Work out the finished part from the listing and answer in its coordinate system (mm). Coordinates: 2 decimals unless noted, no trailing zeros. Order: outer loops, then holes, each group sorted by start corner. A loop starts at its lowest first (then second) coordinate and runs counter-clockwise, first axis right, second up.
1. Flat-ended cylindrical pins translate along their axes: pin 1 Ø0.6 at (x, y) = (-1, -14) entering from -Z; pin 2 Ø1 at (x, y) = (1.5, 1) entering from -Z; pin 3 Ø4 at (x, y) = (1, -3) entering from -Z. Find the tip coordinate at first contact, or state that the pin passes through.
2. The part is cut by section A-A, the plane y = -6.5. Give the vertices of the cut face in (x, z), then the cut area to 3 significant figures.
3. Find the intervals of material crossed by probe 1 along Z at (x, y) = (2.25, 12); probe 2 along Z at (x, y) = (0, 0.5); probe 3 along Y at (x, z) = (-6, 0.15), in increasing order.
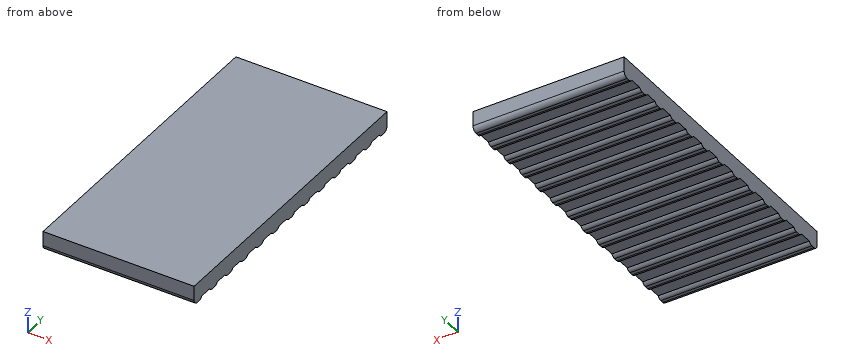
```python
from build123d import *

# Parameters (mm, degrees)
SKETCH1_W           = 15.748
SKETCH1_H           = 31.75
BOSS_EXTRUDE1_DEPTH = 1.778
SKETCH2_W           = 15.748
SKETCH2_H           = 1.27
BOSS_EXTRUDE2_DEPTH = 0.254
FILLET1_R           = 0.508


with BuildPart() as part:
    # Sketch1 → Boss-Extrude1 (new body)
    with BuildSketch(Plane.XY):
        Rectangle(SKETCH1_W, SKETCH1_H)
    extrude(amount=BOSS_EXTRUDE1_DEPTH)

    # Sketch2 → Boss-Extrude2 (add)
    with BuildSketch(Plane(origin=(0, 0, 0), x_dir=(-1, 0, 0), z_dir=(0, 0, -1))):
        with Locations((0, -15.24)):
            Rectangle(SKETCH2_W, SKETCH2_H)
        with Locations((0, -12.7)):
            Rectangle(SKETCH2_W, SKETCH2_H)
        with Locations((0, -10.16)):
            Rectangle(SKETCH2_W, SKETCH2_H)
        with Locations((0, -7.62)):
            Rectangle(SKETCH2_W, SKETCH2_H)
        with Locations((0, -5.08)):
            Rectangle(SKETCH2_W, SKETCH2_H)
        with Locations((0, -2.54)):
            Rectangle(SKETCH2_W, SKETCH2_H)
        Rectangle(SKETCH2_W, SKETCH2_H)
        with Locations((0, 2.54)):
            Rectangle(SKETCH2_W, SKETCH2_H)
        with Locations((0, 5.08)):
            Rectangle(SKETCH2_W, SKETCH2_H)
        with Locations((0, 7.62)):
            Rectangle(SKETCH2_W, SKETCH2_H)
        with Locations((0, 10.16)):
            Rectangle(SKETCH2_W, SKETCH2_H)
        with Locations((0, 12.7)):
            Rectangle(SKETCH2_W, SKETCH2_H)
        with Locations((0, 15.24)):
            Rectangle(SKETCH2_W, SKETCH2_H)
    extrude(amount=BOSS_EXTRUDE2_DEPTH)

    # Fillet1
    # the kernel refuses this fillet: 0.508 mm, written as the material it takes off along each edge
    with BuildSketch(Plane(origin=(9.144, 15.875, -0.254), x_dir=(0, 0, 1), z_dir=(-1, 0, 0))) as fillet1_piece_1:
        with BuildLine():
            CenterArc((FILLET1_R, -FILLET1_R), FILLET1_R, 90, 90)
            Line((0, -FILLET1_R), (-FILLET1_R * 0.02, -FILLET1_R))
            Line((-FILLET1_R * 0.02, -FILLET1_R), (-FILLET1_R * 0.02, FILLET1_R * 0.02))
            Line((-FILLET1_R * 0.02, FILLET1_R * 0.02), (FILLET1_R, FILLET1_R * 0.02))
            Line((FILLET1_R, FILLET1_R * 0.02), (FILLET1_R, 0))
        make_face()
    extrude(amount=18.288, mode=Mode.SUBTRACT)
    with BuildSketch(Plane(origin=(-8.973852263, 14.605, -0.254), x_dir=(0, 0, 1), z_dir=(1, 0, 0)), Plane(origin=(-8.973852263, 12.065, -0.254), x_dir=(0, 0, 1), z_dir=(1, 0, 0)), Plane(origin=(-8.973852263, 9.525, -0.254), x_dir=(0, 0, 1), z_dir=(1, 0, 0)), Plane(origin=(-8.973852263, 6.985, -0.254), x_dir=(0, 0, 1), z_dir=(1, 0, 0)), Plane(origin=(-8.973852263, 4.445, -0.254), x_dir=(0, 0, 1), z_dir=(1, 0, 0)), Plane(origin=(-8.973852263, 1.905, -0.254), x_dir=(0, 0, 1), z_dir=(1, 0, 0)), Plane(origin=(-8.973852263, -0.635, -0.254), x_dir=(0, 0, 1), z_dir=(1, 0, 0)), Plane(origin=(-8.973852263, -3.175, -0.254), x_dir=(0, 0, 1), z_dir=(1, 0, 0)), Plane(origin=(-8.973852263, -5.715, -0.254), x_dir=(0, 0, 1), z_dir=(1, 0, 0)), Plane(origin=(-8.973852263, -8.255, -0.254), x_dir=(0, 0, 1), z_dir=(1, 0, 0)), Plane(origin=(-8.973852263, -10.795, -0.254), x_dir=(0, 0, 1), z_dir=(1, 0, 0)), Plane(origin=(-8.973852263, -13.335, -0.254), x_dir=(0, 0, 1), z_dir=(1, 0, 0))) as fillet1_piece_2:
        with BuildLine():
            CenterArc((0.508, -0.439940905), FILLET1_R, 120, 60)
            Line((0, -0.439940905), (-0.01016, -0.439940905))
            Line((-0.01016, -0.439940905), (-0.01016, 0))
            Line((-0.01016, 0), (0, 0.01016))
            ThreePointArc((0, 0.01016), (0.127, 0.01016), (0.24892, 0.008798818))
            Line((0.24892, 0.008798818), (0.254, 0))
        make_face()
    extrude(amount=17.947704526, mode=Mode.SUBTRACT)
    with BuildSketch(Plane(origin=(8.973852263, 13.335, -0.254), x_dir=(0, -1, 0), z_dir=(-1, 0, 0)), Plane(origin=(8.973852263, 10.795, -0.254), x_dir=(0, -1, 0), z_dir=(-1, 0, 0)), Plane(origin=(8.973852263, 8.255, -0.254), x_dir=(0, -1, 0), z_dir=(-1, 0, 0)), Plane(origin=(8.973852263, 5.715, -0.254), x_dir=(0, -1, 0), z_dir=(-1, 0, 0)), Plane(origin=(8.973852263, 3.175, -0.254), x_dir=(0, -1, 0), z_dir=(-1, 0, 0)), Plane(origin=(8.973852263, 0.635, -0.254), x_dir=(0, -1, 0), z_dir=(-1, 0, 0)), Plane(origin=(8.973852263, -1.905, -0.254), x_dir=(0, -1, 0), z_dir=(-1, 0, 0)), Plane(origin=(8.973852263, -4.445, -0.254), x_dir=(0, -1, 0), z_dir=(-1, 0, 0)), Plane(origin=(8.973852263, -6.985, -0.254), x_dir=(0, -1, 0), z_dir=(-1, 0, 0)), Plane(origin=(8.973852263, -9.525, -0.254), x_dir=(0, -1, 0), z_dir=(-1, 0, 0)), Plane(origin=(8.973852263, -12.065, -0.254), x_dir=(0, -1, 0), z_dir=(-1, 0, 0))) as fillet1_piece_3:
        with BuildLine():
            CenterArc((0.439940905, 0.508), FILLET1_R, 210, 60)
            Line((0, 0.254), (-0.008798818, 0.24892))
            ThreePointArc((-0.008798818, 0.24892), (-0.01016, 0.127), (-0.01016, 0))
            Line((-0.01016, 0), (0, -0.01016))
            Line((0, -0.01016), (0.439940905, -0.01016))
            Line((0.439940905, -0.01016), (0.439940905, 0))
        make_face()
    extrude(amount=17.947704526, mode=Mode.SUBTRACT)
    with BuildSketch(Plane(origin=(9.144, -15.875, -0.254), x_dir=(0, 0, 1), z_dir=(-1, 0, 0))) as fillet1_piece_4:
        with BuildLine():
            CenterArc((FILLET1_R, FILLET1_R), FILLET1_R, 180, 90)
            Line((0, FILLET1_R), (-FILLET1_R * 0.02, FILLET1_R))
            Line((-FILLET1_R * 0.02, FILLET1_R), (-FILLET1_R * 0.02, -FILLET1_R * 0.02))
            Line((-FILLET1_R * 0.02, -FILLET1_R * 0.02), (FILLET1_R, -FILLET1_R * 0.02))
            Line((FILLET1_R, -FILLET1_R * 0.02), (FILLET1_R, 0))
        make_face()
    extrude(amount=18.288, mode=Mode.SUBTRACT)
    with BuildSketch(Plane(origin=(-8.973852263, -14.605, -0.254), x_dir=(0, -1, 0), z_dir=(1, 0, 0))) as fillet1_piece_5:
        with BuildLine():
            CenterArc((0.439940905, -0.508), FILLET1_R, 90, 60)
            Line((0, -0.254), (-0.008798818, -0.24892))
            ThreePointArc((-0.008798818, -0.24892), (-0.01016, -0.127), (-0.01016, 0))
            Line((-0.01016, 0), (0, 0.01016))
            Line((0, 0.01016), (0.439940905, 0.01016))
            Line((0.439940905, 0.01016), (0.439940905, 0))
        make_face()
    extrude(amount=17.947704526, mode=Mode.SUBTRACT)


solid = part.part
```
Geometry says:
1. pin 1: stops at z = 0
1. pin 2: stops at z = -0.15
1. pin 3: stops at z = -0.25
2. outline: (-7.87, 0) - (7.87, 0) - (7.87, 1.78) - (-7.87, 1.78) - close
2. area: 28.0 mm2
3. probe 1: z = 0 to 1.78
3. probe 2: z = -0.15 to 1.78
3. probe 3: y = -15.86 to 15.86
